Model file for the job. Use its own axes, mm. Face numbers are marked on the shaded views. A direction names the side the tool comes from. Round coordinates to 2 decimals unless told otherwise and drop trailing zeros. Order: outer loops, then holes, each group sorted by start corner. A loop starts at its lowest first (then second) coordinate and runs counter-clockwise, first axis right, second up. Notation, with made-up numbers: (12, -10.5) -> (68, -10.5) arc R12 ccw to (68, 12.5) -> close; hole circle Ø5 at (49, 56.25). An arc over 180 degrees is marked (long way). Answer as CSV lines item,"result".
```python
from build123d import *

# Parameters (mm, degrees)
F0_W     = 100
F0_H     = 100
F1_DEPTH = 2
F2_W     = 2
F2_H     = 2
F2_W_2   = 8
F2_H_2   = 10
F3_DEPTH = 10


with BuildPart() as f1:
    # F0 (on Top) → F1 (new body)
    with BuildSketch(Plane.XY):
        Rectangle(F0_W, F0_H)
    extrude(amount=F1_DEPTH)

    # F2 (on face) → F3 (join)
    with BuildSketch(Plane.XY.offset(2)):
        Polygon((-48, 50), (-50, 50), (-50, -30), (-48, -30), (-48, 10), (-48, 12), (-48, 40), (-48, 42), align=None)
        with Locations((-49, -31)):
            Rectangle(F2_W, F2_H)
        with Locations((-44, 41)):
            Rectangle(F2_W_2, F2_H)
        Polygon((-48, -32), (-50, -32), (-50, -50), (-48, -50), (-48, -48.655497), align=None)
        with Locations((-44, -31)):
            Rectangle(F2_W_2, F2_H)
        Polygon((-48, 12), (-48, 10), (-20, 10), (-20, 38), (-12, 38), (-12, 40), (-22, 40), (-22, 12), align=None)
        Polygon((-48, -48.655497), (-48, -50), (40, -50), (40, -48.655497), (18.924282, -48.655497), (13.644133, -48.655497), align=None)
        Polygon((22.337581, -38.566588), (13.644133, -48.655497), (18.924282, -48.655497), (25.367798, -41.177677), align=None)
        Polygon((48, -15.875603), (48, -50), (50, -50), (50, 50), (-30, 50), (-30, 48), (48, 48), (48, -8.784876), align=None)
        Polygon((47.523779, -15.465251), (48, -15.875603), (48, -8.784876), (27.559759, -32.506154), (30.589976, -35.117243), align=None)
        Polygon((-30, 48), (-30, 50), (-32, 50), (-32, 48), (-32, 22), (-38, 22), (-40, 22), (-40, 20), (-30, 20), align=None)
        with Locations((-36, 49)):
            Rectangle(F2_W_2, F2_H)
        with Locations((-39, 27)):
            Rectangle(F2_W, F2_H_2)
    extrude(amount=F3_DEPTH)


solid = f1.part
```
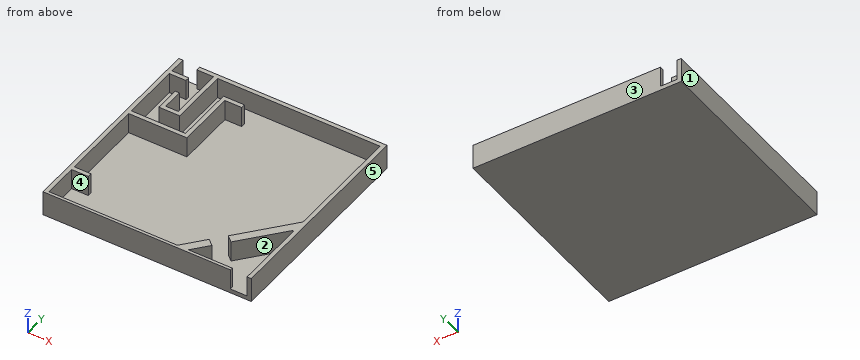
Q1. Mould opens along X. For the marked faces 1, 2 and 3 say: +X half, -X half, draft (parallel to the pull), parting line (faces both ways), or undercut.
Checks:
face 1,"-X half"
face 2,"undercut"
face 3,"draft"
Q2. Saw through at C-C (y = 36). Write the cut outline in (x, z).
Checks:
outline,"(-50, 0) -> (50, 0) -> (50, 12) -> (48, 12) -> (48, 2) -> (-20, 2) -> (-20, 12) -> (-22, 12) -> (-22, 2) -> (-30, 2) -> (-30, 12) -> (-32, 12) -> (-32, 2) -> (-48, 2) -> (-48, 12) -> (-50, 12) -> close"
Q3. Saw through at D-D (x = 33.5). Write the cut outline in (y, z).
Checks:
outline,"(-50, 0) -> (50, 0) -> (50, 12) -> (48, 12) -> (48, 2) -> (-25.61, 2) -> (-25.61, 12) -> (-31.74, 12) -> (-31.74, 2) -> (-48.66, 2) -> (-48.66, 12) -> (-50, 12) -> close"
Q4. Wall check: L1, parallel to Y at x = -25, z = 3.75; L2, parallel to X at y = 41.5, z = 7; L3, parallel to X at y = 26.5, z = 3. Give the ranges that are in metal, low to high. Write a range as [from, to].
Checks:
L1,"[-50, -48.66], [10, 12], [48, 50]"
L2,"[-50, -40], [-32, -30], [48, 50]"
L3,"[-50, -48], [-40, -38], [-32, -30], [-22, -20], [48, 50]"
Q5. Saw through at B-B (x = 2.5). Write the cut outline in (y, z).
Checks:
outline,"(-50, 0) -> (50, 0) -> (50, 12) -> (48, 12) -> (48, 2) -> (-48.66, 2) -> (-48.66, 12) -> (-50, 12) -> close"
Q6. Tool access for the marked faces 4 and 5: list every direction of +Z, -Z, +X, -X, +Y, -Y with a clear straight run to the whole face (end or side of a thin tool).
Checks:
face 4,"+Z"
face 5,"+Z, -Z, +X, +Y, -Y"
Q7. Saw through at A-A (y = 8.5). Write the cut outline in (x, z), plus the area to 3 significant figures.
Checks:
outline,"(-50, 0) -> (50, 0) -> (50, 12) -> (48, 12) -> (48, 2) -> (-48, 2) -> (-48, 12) -> (-50, 12) -> close"
area,"240 mm²"
